Geometry: final body of the model. Coordinates: model frame, mm. A direction names the side the tool comes from. Round coordinates to 2 decimals unless told otherwise and drop trailing zeros. Loops run counter-clockwise (first coordinate to the right, second up) from the corner with the lowest first, then second, coordinate; pieces in that order, holes last. Notation, with made-up numbers: (4.25, 83.5) - (15.25, 83.5) arc R24 ccw to (15.25, 96.5) - close; hole circle Ø2 at (45.25, 84). An arc over 180 degrees is marked (long way). Answer as a JSON object with one key per item and string values. Group by question number.
Item 1: Section B-B (x = -65). Return the cut outline in (y, z).
Item 2: Section A-A (y = 47). Count the separate pieces of the cut face and the enclosed holes in it, plus the area to 3 significant figures.
Item 3: First-contact query: pin 1 (25 mm diameter, centred on x = 207, y = 69.5, fed in from +Z); pin 2 (22.5 mm diameter, centred on y = 106.5, z = -149.5, fed in from -X); pin 3 (15 mm diameter, centred on x = 198, y = 66, fed in from -Z). Flat tips, straight axial feed; report the tip coordinate or a pass-through.
Item 4: Section C-C (y = 139). Return the cut outline in (x, z).
Item 5: Line query: line 1 (Z direction, x = 62.5, y = 13); line 2 (Y direction, x = 95, z = -193.5); line 3 (Y direction, x = 193.5, z = 108.5). Output: solid intervals per line, ascending.
Item 6: Draft query along Y for faces 6 (the face through (92.83, 37.24, 195.07)), 7 (the face through (54, 180, 192)), 8 (the face through (-3, 89, -190)). Return one class per face: released by +Y, released by -Y, zero draft, split by the parting line, or undercut.
Item 7: Section D-D (z = 142). Return the cut outline in (x, y), plus the area to 3 significant figures.
Item 8: Reachability of faces 1 (the face through (175, 89, -162)), 2 (the face through (-3, 89, 190)), 3 (the face through (-2, 89, 200)), 4 (the face through (175, 89, 163)), 5 (the face through (195, 89, -115)) from +Z, -Z, +X, -X, +Y, -Y: full face, straight path, thin tool, end or side. Return the list, or none.
```python
from build123d import *

# Parameters (mm, degrees)
SKETCH1_W           = 350
SKETCH1_H           = 400
SKETCH1_W_2         = 50
SKETCH1_H_2         = 250
BOSS_EXTRUDE1_DEPTH = 180
CUT_EXTRUDE1_DEPTH  = 179
SKETCH3_W           = 230
SKETCH3_H           = 179
CUT_EXTRUDE2_DEPTH  = 10
SKETCH4_W           = 380
SKETCH4_H           = 179
CUT_EXTRUDE3_DEPTH  = 10
SKETCH5_R           = 10
CUT_EXTRUDE4_DEPTH  = 401


with BuildPart() as part:
    # Sketch1 → Boss-Extrude1 (new body)
    with BuildSketch(Plane(origin=(0, 0, 0), x_dir=(1, 0, 0), z_dir=(0, 1, 0))):
        Rectangle(SKETCH1_W, SKETCH1_H)
        with Locations((200, 0)):
            Rectangle(SKETCH1_W_2, SKETCH1_H_2)
    extrude(amount=BOSS_EXTRUDE1_DEPTH)

    # Sketch2 → Cut-Extrude1 (cut)
    with BuildSketch(Plane(origin=(0, 180, 0), x_dir=(1, 0, 0), z_dir=(0, 1, 0))):
        Polygon((215, 115), (165, 115), (165, 190), (-165, 190), (-165, -190), (165, -190), (165, -115), (215, -115), align=None)
    extrude(amount=-CUT_EXTRUDE1_DEPTH, mode=Mode.SUBTRACT)

    # Sketch3 → Cut-Extrude2 (cut)
    with BuildSketch(Plane.ZY.offset(-215)):
        with Locations((0, 90.5)):
            Rectangle(SKETCH3_W, SKETCH3_H)
    extrude(amount=-CUT_EXTRUDE2_DEPTH, mode=Mode.SUBTRACT)

    # Sketch4 → Cut-Extrude3 (cut)
    with BuildSketch(Plane(origin=(-165, 0, 0), x_dir=(0, 0, -1), z_dir=(1, 0, 0))):
        with Locations((0, 90.5)):
            Rectangle(SKETCH4_W, SKETCH4_H)
    extrude(amount=-CUT_EXTRUDE3_DEPTH, mode=Mode.SUBTRACT)

    # Sketch5 → Cut-Extrude4 (cut, through all)
    with BuildSketch(Plane.XY.offset(200)):
        with Locations((95, 47)):
            Circle(SKETCH5_R)
        with Locations((-65, 47)):
            Circle(SKETCH5_R)
    extrude(amount=-CUT_EXTRUDE4_DEPTH, mode=Mode.SUBTRACT)


solid = part.part
```
Values:
{
 "1": {"outline": "(0, -200) - (37, -200) - (37, -190) - (1, -190) - (1, 190) - (37, 190) - (37, 200) - (0, 200) - close; (57, -200) - (180, -200) - (180, -190) - (57, -190) - close; (57, 190) - (180, 190) - (180, 200) - (57, 200) - close"},
 "2": {"separate pieces": "6", "enclosed holes": "0", "area": "8,700 mm^2"},
 "3": {"pin 1": "stops at z = 125", "pin 2": "stops at x = 165", "pin 3": "stops at z = -125"},
 "4": {"outline": "(-175, -200) - (175, -200) - (175, -125) - (225, -125) - (225, -115) - (165, -115) - (165, -190) - (-175, -190) - close; (-175, 190) - (165, 190) - (165, 115) - (225, 115) - (225, 125) - (175, 125) - (175, 200) - (-175, 200) - close"},
 "5": {"line 1": "z = -200 to -190, 190 to 200", "line 2": "y = 0 to 37, 57 to 180", "line 3": "y = 0 to 1"},
 "6": {"face 6": "undercut", "face 7": "released by +Y", "face 8": "zero draft"},
 "7": {"outline": "(-175, 0) - (175, 0) - (175, 180) - (165, 180) - (165, 1) - (-175, 1) - close", "area": "2,140 mm^2"},
 "8": {"face 1": "-Z, +X, +Y, -Y", "face 2": "-X, +Y", "face 3": "+Z, +X, -X, +Y, -Y", "face 4": "+Z, +X, +Y, -Y", "face 5": "+X, -X, +Y"}
}
